Can you work these out from the model? Positions are in its coordinate system, mm. Face numbers are marked on the shaded views. A direction names the side the tool comes from. Coordinates: 2 decimals unless noted, no trailing zeros. Write each loop counter-clockwise with the first axis right and the second up, starting at its lowest first coordinate (ties: lowest second). Pieces come first, ordered by that corner, then holes. Notation, with made-up numbers: (77, 85) -> (115, 85) arc R27 ccw to (115, 102) -> close; hole circle Ø6 at (71.25, 18.25). An arc over 180 degrees is marked (long way). Use one line per item in the form item = value.
```python
from build123d import *

# Parameters (mm, degrees)
SKETCH1_W           = 58
SKETCH1_H           = 20
BOSS_EXTRUDE1_DEPTH = 3
SKETCH2_R           = 2.210718461
SKETCH2_R_2         = 2.399764385
SKETCH2_R_3         = 2.478849081
SKETCH2_R_4         = 2.403854655
CUT_EXTRUDE1_DEPTH  = 10
SKETCH3_W           = 41.706821958
SKETCH3_H           = 20
BOSS_EXTRUDE2_DEPTH = 7
SKETCH4_R           = 3.15
CUT_EXTRUDE2_DEPTH  = 20
SKETCH5_R           = 0.5
CUT_EXTRUDE3_DEPTH  = 22


with BuildPart() as part:
    # Sketch1 → Boss-Extrude1 (new body)
    with BuildSketch(Plane(origin=(0, 0, 0), x_dir=(1, 0, 0), z_dir=(0, 1, 0))):
        with Locations((29, 10)):
            Rectangle(SKETCH1_W, SKETCH1_H)
    extrude(amount=BOSS_EXTRUDE1_DEPTH)

    # Sketch2 → Cut-Extrude1 (cut)
    with BuildSketch(Plane(origin=(0, 3, 0), x_dir=(1, 0, 0), z_dir=(0, 1, 0))):
        with Locations(Location((54.154962959, 14.898762514, 0), (0, 0, 270))):
            Circle(SKETCH2_R)
        with Locations(Location((54.154962959, 4.898762514, 0), (0, 0, 270))):
            Circle(SKETCH2_R_2)
        with Locations(Location((4.375736357, 4.898762514, 0), (0, 0, 270))):
            Circle(SKETCH2_R_3)
        with Locations(Location((4.375736357, 14.898762514, 0), (0, 0, 270))):
            Circle(SKETCH2_R_4)
    extrude(amount=-CUT_EXTRUDE1_DEPTH, mode=Mode.SUBTRACT)

    # Sketch3 → Boss-Extrude2 (add)
    with BuildSketch(Plane.XZ):
        with Locations((29.286245635, -10)):
            Rectangle(SKETCH3_W, SKETCH3_H)
    extrude(amount=BOSS_EXTRUDE2_DEPTH)

    # Sketch4 → Cut-Extrude2 (cut)
    with BuildSketch(Plane(origin=(0, 3, 0), x_dir=(1, 0, 0), z_dir=(0, 1, 0))):
        with Locations(Location((39.565349658, 10, 0), (0, 0, 270))):
            Circle(SKETCH4_R)
    extrude(amount=-CUT_EXTRUDE2_DEPTH, mode=Mode.SUBTRACT)

    # Sketch5 → Cut-Extrude3 (cut)
    with BuildSketch(Plane.XZ.offset(7)):
        with Locations(Location((26.035349658, -10, 0), (0, 0, 270))):
            Circle(SKETCH5_R)
        with Locations(Location((29.035349658, -10, 0), (0, 0, 270))):
            Circle(SKETCH5_R)
        with Locations(Location((23.035349658, -10, 0), (0, 0, 270))):
            Circle(SKETCH5_R)
        with Locations(Location((32.035349658, -10, 0), (0, 0, 270))):
            Circle(SKETCH5_R)
        with Locations(Location((47.095349658, -10, 0), (0, 0, 270))):
            Circle(SKETCH5_R)
    extrude(amount=-CUT_EXTRUDE3_DEPTH, mode=Mode.SUBTRACT)


solid = part.part
```
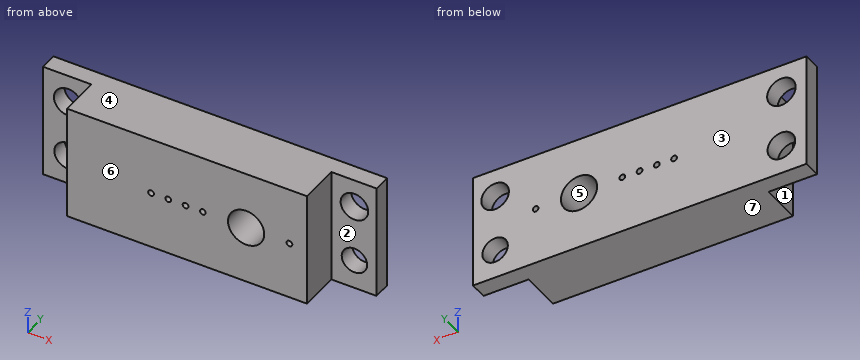
Q1. Suppose I cut it at D-D (z = -19). Write out the boundary of the cut face in (x, y), then the cut area to 3 significant figures.
Return value:
outline = (0, 0) -> (8.43, 0) -> (8.43, -7) -> (50.14, -7) -> (50.14, 0) -> (58, 0) -> (58, 3) -> (0, 3) -> close
area = 466 mm2
Q2. Suppose I cut it at B-B (z = -14.75). Write out the boundary of the cut face in (x, y).
Return value:
outline = (0, 0) -> (1.98, 0) -> (1.98, 3) -> (0, 3) -> close; (6.77, 0) -> (8.43, 0) -> (8.43, -7) -> (50.14, -7) -> (50.14, 0) -> (51.95, 0) -> (51.95, 3) -> (6.77, 3) -> close; (56.36, 0) -> (58, 0) -> (58, 3) -> (56.36, 3) -> close
Q3. Suppose I cut it at A-A (z = -10). Give the number of separate pieces and of enclosed holes in the cut face, then the cut area to 3 significant figures.
Return value:
separate_pieces = 7
enclosed_holes = 0
area = 353 mm2
Q4. Thinking about a two-plate mould opening in Z: for the marked faces 4, 5, 6 and 7, which applies, released by +Z, released by -Z, zero draft, split by the parting line, or undercut?
Return value:
face_4 = released by +Z
face_5 = undercut
face_6 = zero draft
face_7 = released by -Z
Q5. For the marked faces 1, 2 and 3, which set-ups out of +Z, -Z, +X, -X, +Y, -Y let a thin tool reach every point of the face, with its end or its side?
Return value:
face_1 = +Z, -Z, -X, -Y
face_2 = +Z, -Z, +X, -Y
face_3 = +Z, -Z, +X, -X, +Y
Q6. If I drill on line 1 (X direction, y = -5, z = -1.25); line 2 (Z direction, x = 39, y = -2); line 3 (X direction, y = -2.75, z = -8.75), over which ranges is the centre line in solid material (lowest first)? Write a range as from..to.
Return value:
line_1 = 8.43..50.14
line_2 = -20..-13.1, -6.9..0
line_3 = 8.43..36.67, 42.46..50.14
Q7. Will these pins go through, and if not, where does the flat tip stop? pin 1 (7 mm diameter, centred on x = 54.15, z = -14.9, fed in from -Y); pin 2 (1.5 mm diameter, centred on y = -5, z = -16, fed in from -X).
Return value:
pin_1 = 0
pin_2 = 8.43
